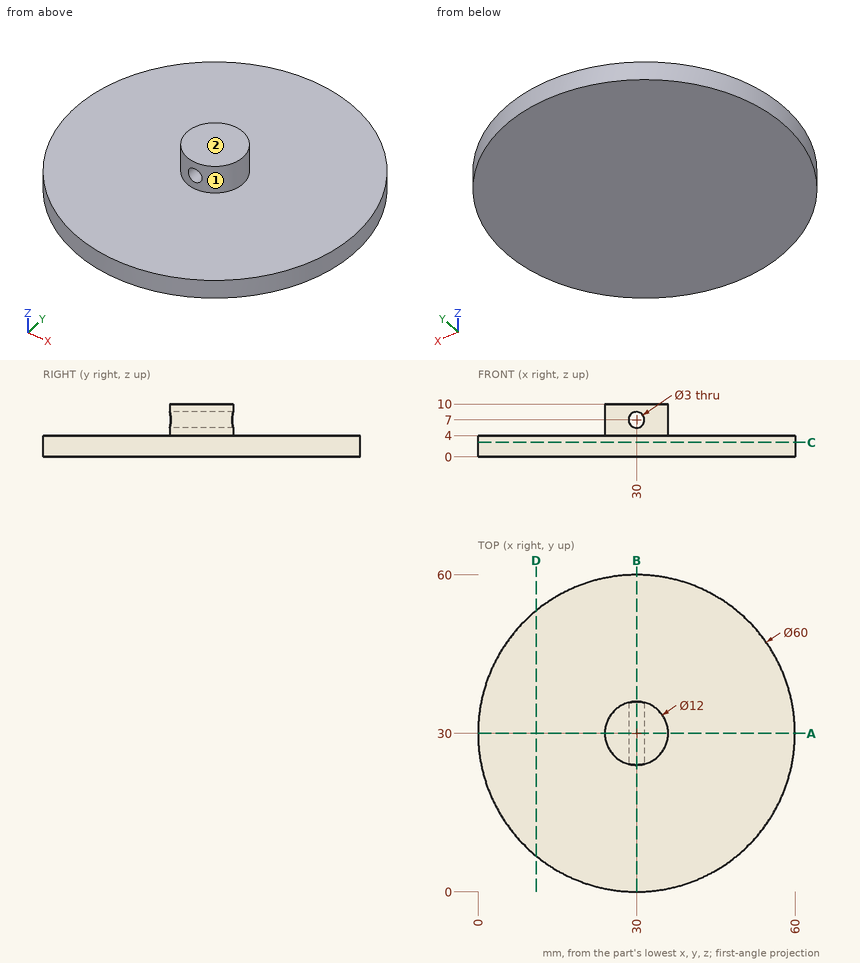
Geometry check sheet. Reference: drawing and pictorial views, mm from the part's lowest x, y, z. A direction names the side the tool comes from. Round coordinates to 2 decimals unless told otherwise and drop trailing zeros. Loops run counter-clockwise (first coordinate to the right, second up) from the corner with the lowest first, then second, coordinate; pieces in that order, holes last. Notation, with made-up numbers: (10.25, 48) -> (47.25, 48) arc R7 cw to (47.25, 54) -> close; hole circle Ø3 at (5.5, 74.25). An arc over 180 degrees is marked (long way). Answer as a JSON object with one key per item and string values.
Q1. Section check C-C (z = 2.75). Record the boundary of the cut face in (x, y).
Data:
{"outline": "circle Ø60 at (30, 30)"}
Q2. Section check D-D (x = 11). Record the boundary of the cut face in (y, z).
Data:
{"outline": "(6.78, 0) -> (53.22, 0) -> (53.22, 4) -> (6.78, 4) -> close"}
Q3. Scan lines: line 1 (Z direction, x = 30, y = 30.75); line 2 (Z direction, x = 53, y = 11); line 3 (X direction, y = 28, z = 7). Record each from-to range of solid material in increasing order. Write a range as from..to.
Data:
{"line 1": "z = 0..5.5, 8.5..10", "line 2": "z = 0..4", "line 3": "x = 24.34..28.5, 31.5..35.66"}
Q4. Access from +Z, -Z, +X, -X, +Y, -Y to the whole of each face (thin tool, end or side, straight path). Record for the marked faces 1 and 2.
Data:
{"face 1": "+Z", "face 2": "+Z, +X, -X, +Y, -Y"}
Q5. Section check A-A (y = 30). Record the boundary of the cut face in (x, z), then the cut area to 3 significant figures.
Data:
{"outline": "(0, 0) -> (60, 0) -> (60, 4) -> (36, 4) -> (36, 10) -> (24, 10) -> (24, 4) -> (0, 4) -> close; hole circle Ø3 at (30, 7)", "area": "305 mm2"}
Q6. Go/stop test with flat-tipped pins: P1, Ø3, axis at x = 11.5, y = 11.5, coming from the +Z side; P2, Ø3, axis at y = 50, z = 4.5, coming from the +X side; P3, Ø3, axis at y = 51, z = 5, coming from the -X side. Record where each tip stops, or that it passes through.
Data:
{"P1": "stops at z = 4", "P2": "stops at x = 53.55", "P3": "stops at x = 7.53"}
Q7. Section check B-B (x = 30). Record the boundary of the cut face in (y, z), then the cut area to 3 significant figures.
Data:
{"outline": "(0, 0) -> (60, 0) -> (60, 4) -> (36, 4) -> (36, 5.5) -> (24, 5.5) -> (24, 4) -> (0, 4) -> close; (24, 8.5) -> (36, 8.5) -> (36, 10) -> (24, 10) -> close", "area": "276 mm2"}
